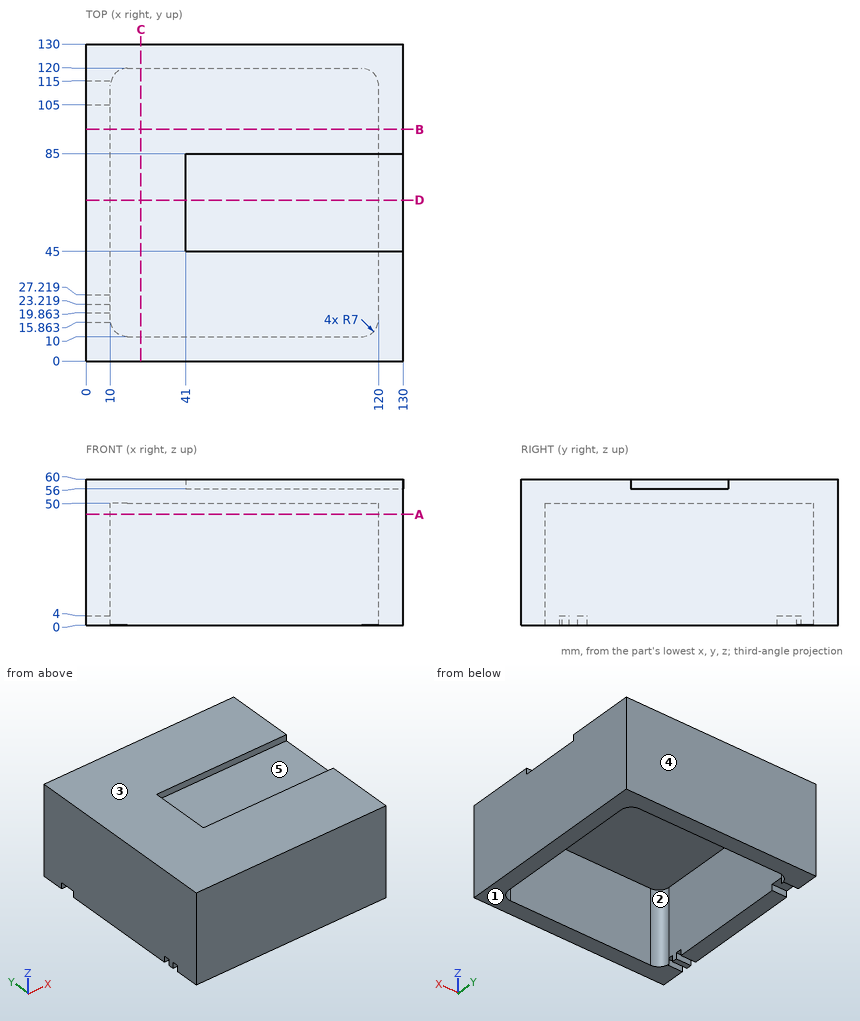
Input: dimensioned drawing with shaded views. Units: mm. Origin: part minimum x, y, z. A direction names the side the tool comes from. Round coordinates to 2 decimals unless told otherwise and drop trailing zeros. Order: outer loops, then holes, each group sorted by start corner. A loop starts at its lowest first (then second) coordinate and runs counter-clockwise, first axis right, second up. Notation, with made-up numbers: (10, 9.25) -> (50, 9.25) arc R10 cw to (50, 19.25) -> close; hole circle Ø7 at (-25, 43). An arc over 180 degrees is marked (long way). One line per item, written item: value. Start each with the question number.
Q1. Section query B-B (y = 95). Return the cut outline in (x, z), plus the area to 3 significant figures.
Q2. Pin query (flat end, axial travel): pin 1 (1.2 mm diameter, centred on x = 4, y = 24.5, fed in from -Z); pin 2 (4 mm diameter, centred on x = 95.5, y = 23, fed in from -Z); pin 3 (12 mm diameter, centred on x = 66.5, y = 63.5, fed in from +Z). Return the tip coordinate at first contact, or that it passes through.
Q3. Section query A-A (z = 45.5). Return the cut outline in (x, y).
Q4. Draft query along Y for the marked faces 3, 4 and 5. Return one class per face: pulls with the +Y half, pulls with the -Y half, needs draft (parallel to the pull), parting line crosses it, or undercut.
Q5. Access query for the marked faces 1 and 2. Directions: +Z, -Z, +X, -X, +Y, -Y. A direction counts if a zero-diameter tool reaches every point of the face in a straight line with its end or side. Return the directions, or none.
Q6. Material intervals for probe 1 along X at (y, z) = (97.5, 7); probe 2 along Z at (x, y) = (50, 20.5), sorted ascending.
Q7. Section query D-D (y = 66). Return the cut outline in (x, z).
Findings below:
1. outline: (0, 0) -> (10, 0) -> (10, 50) -> (120, 50) -> (120, 0) -> (130, 0) -> (130, 60) -> (0, 60) -> close
1. area: 2,300 mm²
2. pin 1: z = 4
2. pin 2: z = 50
2. pin 3: z = 56
3. outline: (0, 0) -> (130, 0) -> (130, 130) -> (0, 130) -> close; hole (10, 17) arc R7 ccw to (17, 10) -> (113, 10) arc R7 ccw to (120, 17) -> (120, 113) arc R7 ccw to (113, 120) -> (17, 120) arc R7 ccw to (10, 113) -> close
4. face 3: needs draft
4. face 4: pulls with the +Y half
4. face 5: undercut
5. face 1: -Z, +X, -X, +Y, -Y
5. face 2: -Z
6. probe 1: 0 to 10, 120 to 130
6. probe 2: 50 to 60
7. outline: (0, 0) -> (10, 0) -> (10, 50) -> (120, 50) -> (120, 0) -> (130, 0) -> (130, 56) -> (41, 56) -> (41, 60) -> (0, 60) -> close
